```python
from build123d import *

# Parameters (mm, degrees)
SLEEVE_OUTLINE_DEPTH = 46
SKETCH2_4_W          = 6.825
SKETCH2_4_H          = 90
BEAM_MOUNTING_DEPTH  = 40
SKETCH3_R            = 1.75
NUT_INSERTS_DEPTH    = 3
SKETCH3_4_R          = 1.75
SCREW_INSERTS_DEPTH  = 23
SKETCH4_R            = 1.55
BOARD_SHAPING_DEPTH  = 10


with BuildPart() as part:
    # Sketch2 → Sleeve_Outline (new body)
    with BuildSketch(Plane.XY):
        Polygon((-14.5875, 90), (0, 90), (6.825, 90), (10, 90), (10.005, 90), (13.005, 90), (31.4125, 90), (31.4125, 95), (-14.5875, 95), align=None)
    extrude(amount=SLEEVE_OUTLINE_DEPTH)

    # Sketch2<4> → Beam_Mounting (add)
    with BuildSketch(Plane.XY):
        with Locations((3.4125, 45)):
            Rectangle(SKETCH2_4_W, SKETCH2_4_H)
        Polygon((10.005, 90), (13.005, 90), (10.005, 87), align=None)
    extrude(amount=BEAM_MOUNTING_DEPTH)

    # Sketch3 → Nut_Inserts (cut)
    # profile 1 of 6: a face of its own
    with BuildSketch(Plane(origin=(6.825, 0, 0), x_dir=(0, 0, -1), z_dir=(1, 0, 0))):
        Polygon((-30, 45), (-31.875, 48.247595264), (-35.625, 48.247595264), (-37.5, 45), (-35.625, 41.752404736), (-31.875, 41.752404736), align=None)
        with Locations((-33.75, 45)):
            Circle(SKETCH3_R, mode=Mode.SUBTRACT)
    # profile 2 of 6: a face of its own
    with BuildSketch(Plane(origin=(6.825, 0, 0), x_dir=(0, 0, -1), z_dir=(1, 0, 0))):
        Polygon((-37.5, 22.5), (-35.625, 19.252404736), (-31.875, 19.252404736), (-30, 22.5), (-31.875, 25.747595264), (-35.625, 25.747595264), align=None)
        with Locations((-33.75, 22.5)):
            Circle(SKETCH3_R, mode=Mode.SUBTRACT)
    # profile 3 of 6: a face of its own
    with BuildSketch(Plane(origin=(6.825, 0, 0), x_dir=(0, 0, -1), z_dir=(1, 0, 0))):
        Polygon((-37.5, 67.5), (-35.625, 64.252404736), (-31.875, 64.252404736), (-30, 67.5), (-31.875, 70.747595264), (-35.625, 70.747595264), align=None)
        with Locations((-33.75, 67.5)):
            Circle(SKETCH3_R, mode=Mode.SUBTRACT)
    # profile 4 of 6: a face of its own
    with BuildSketch(Plane(origin=(6.825, 0, 0), x_dir=(0, 0, -1), z_dir=(1, 0, 0))):
        Polygon((-8.125, 70.747595264), (-4.375, 70.747595264), (-2.5, 67.5), (-4.375, 64.252404736), (-8.125, 64.252404736), (-10, 67.5), align=None)
        with Locations((-6.25, 67.5)):
            Circle(SKETCH3_R, mode=Mode.SUBTRACT)
    # profile 5 of 6: a face of its own
    with BuildSketch(Plane(origin=(6.825, 0, 0), x_dir=(0, 0, -1), z_dir=(1, 0, 0))):
        Polygon((-4.375, 48.247595264), (-2.5, 45), (-4.375, 41.752404736), (-8.125, 41.752404736), (-10, 45), (-8.125, 48.247595264), align=None)
        with Locations((-6.25, 45)):
            Circle(SKETCH3_R, mode=Mode.SUBTRACT)
    # profile 6 of 6: a face of its own
    with BuildSketch(Plane(origin=(6.825, 0, 0), x_dir=(0, 0, -1), z_dir=(1, 0, 0))):
        Polygon((-4.375, 25.747595264), (-2.5, 22.5), (-4.375, 19.252404736), (-8.125, 19.252404736), (-10, 22.5), (-8.125, 25.747595264), align=None)
        with Locations((-6.25, 22.5)):
            Circle(SKETCH3_R, mode=Mode.SUBTRACT)
    extrude(amount=-NUT_INSERTS_DEPTH, mode=Mode.SUBTRACT)

    # Sketch3<4> → Screw_Inserts (cut)
    with BuildSketch(Plane(origin=(6.825, 0, 0), x_dir=(0, 0, -1), z_dir=(1, 0, 0))):
        with Locations((-33.75, 67.5)):
            Circle(SKETCH3_4_R)
        with Locations((-33.75, 45)):
            Circle(SKETCH3_4_R)
        with Locations((-33.75, 22.5)):
            Circle(SKETCH3_4_R)
        with Locations((-6.25, 22.5)):
            Circle(SKETCH3_4_R)
        with Locations((-6.25, 45)):
            Circle(SKETCH3_4_R)
        with Locations((-6.25, 67.5)):
            Circle(SKETCH3_4_R)
    extrude(amount=-SCREW_INSERTS_DEPTH, mode=Mode.SUBTRACT)

    # Sketch4 → Board_Shaping (cut)
    with BuildSketch(Plane(origin=(0, 95, 0), x_dir=(1, 0, 0), z_dir=(0, 1, 0))):
        with BuildLine():
            ThreePointArc((-11.5875, -46), (-13.708820344, -45.121320344), (-14.5875, -43))
            Line((-14.5875, -43), (-14.5875, -46))
            Line((-14.5875, -46), (-11.5875, -46))
        make_face()
        with Locations(Location((-11.5875, -43, 0), (0, 0, 270))):
            Circle(SKETCH4_R)
        with Locations(Location((-11.5875, -3, 0), (0, 0, 270))):
            Circle(SKETCH4_R)
        with BuildLine():
            ThreePointArc((-14.5875, -3), (-13.708820344, -0.878679656), (-11.5875, 0))
            Line((-11.5875, 0), (-14.5875, 0))
            Line((-14.5875, 0), (-14.5875, -3))
        make_face()
        with BuildLine():
            Line((31.4125, 0), (28.4125, 0))
            ThreePointArc((28.4125, 0), (30.533820344, -0.878679656), (31.4125, -3))
            Line((31.4125, -3), (31.4125, 0))
        make_face()
        with Locations(Location((28.4125, -3, 0), (0, 0, 270))):
            Circle(SKETCH4_R)
        with Locations(Location((28.4125, -43, 0), (0, 0, 270))):
            Circle(SKETCH4_R)
        with BuildLine():
            Line((31.4125, -46), (31.4125, -43))
            ThreePointArc((31.4125, -43), (30.533820344, -45.121320344), (28.4125, -46))
            Line((28.4125, -46), (31.4125, -46))
        make_face()
    extrude(amount=-BOARD_SHAPING_DEPTH, mode=Mode.SUBTRACT)


solid = part.part
```
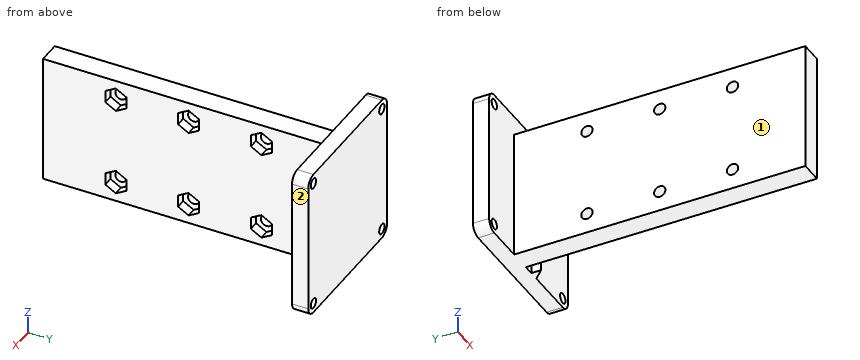
Could you check a few things on this model? Use its own coordinates, in mm. Face numbers are marked on the shaded views. A direction names the side the tool comes from. Give positions to 0.01 mm unless a question says otherwise; leave off trailing zeros. Order: outer loops, then holes, each group sorted by start corner. A loop starts at its lowest first (then second) coordinate and runs counter-clockwise, first axis right, second up.
Q1. For the marked faces 1 and 2, which set-ups out of +Z, -Z, +X, -X, +Y, -Y let a thin tool reach every point of the face, with its end or its side?
Q2. I'm going to push flat-ended pins straight in: P1, Ø4, axis at y = 45, z = 33.75, coming from the -X side; P2, Ø3, axis at y = 22.5, z = 33.75, coming from the +X side; P3, Ø0.9, axis at x = 11, y = 89, coming from the +Z side; P4, Ø5, axis at x = 28.41, z = 43, coming from the -Y side. Where does each tip first touch, or does it pass through?
Q3. Suppose I cut it at A-A, the plane z = 26. Write out the boundary of the cut face in (x, y) (1 decimal).
Q4. If I drill on line 1 along Y through (x, z) = (2.4, 6.25); line 2 along Y through (x, z) = (2, 33); line 3 along X through (y, z) = (65.5, 14.5) (3 decimals), over which ranges is the centre line in solid material (lowest first)?
Q5. Suppose I cut it at D-D, the plane y = 84.5. Write out the boundary of the cut face in (x, z) (3 decimals).
Q6. Suppose I cut it at B-B, the plane z = 33.75. Count the separate pieces of the cut face and the enclosed holes in it, and give its area (3 significant figures).
Q7. Suppose I cut it at C-C, the plane x = 14. Write out the boundary of the cut face in (y, z), and give its area (3 significant figures).
Solution:
1. face 1: +Z, -Z, -X, -Y
1. face 2: +Z, -Z, +X, +Y, -Y
2. P1: stops at x = 0
2. P2: passes through
2. P3: stops at z = 40
2. P4: stops at y = 90
3. outline: (-14.6, 90) - (0, 90) - (0, 0) - (6.8, 0) - (6.8, 90) - (10, 90) - (10, 87) - (13, 90) - (31.4, 90) - (31.4, 95) - (-14.6, 95) - close
4. line 1: y = 0 to 20.75, 24.25 to 43.25, 46.75 to 65.75, 69.25 to 95
4. line 2: y = 0 to 20.92, 24.08 to 43.42, 46.58 to 65.92, 69.08 to 95
4. line 3: x = 0 to 6.825
5. outline: (0, 0) - (6.825, 0) - (6.825, 40) - (0, 40) - close
6. separate pieces: 4
6. enclosed holes: 0
6. area: 750 mm2
7. outline: (90, 0) - (95, 0) - (95, 46) - (90, 46) - close
7. area: 230 mm2
